Autodesk Inventor part; units mm, degrees
ref_plane "YZ Plane" through (0, 0, 0) normal (1, 0, 0) x (0, 1, 0)
ref_plane "XZ Plane" through (0, 0, 0) normal (0, 1, 0) x (-1, 0, 0)
ref_plane "XY Plane" through (0, 0, 0) normal (0, 0, 1) x (1, 0, 0)
sketch "Sketch2" plane through (0, 0, 0) normal (0, 0, 1) x (1, 0, 0)
  circle A0 centre (0, 0) radius 80.5
  circle A1 centre (0, 0) radius 142.5
  dimension "d25" = 161
  dimension "d27" = 285
extrude "Plate2" add sketch "Sketch2" along normal blind 8 contours A0 | A1
sketch "Sketch3" plane through (0, 0, 8) normal (0, 0, 1) x (1, 0, 0)
  circle A0 centre (-120, 0) radius 8.5
  circle A1 centre (0, 0) radius 120 construction
  dimension "d28" = 240
  dimension "d15" = 17
extrude "Cut1" cut sketch "Sketch3" against normal blind 8
pattern_circular "Circular Pattern1" count 8 over 360 about axis through (0, 0, -10) along (0, 0, 1) of "Cut1"
equation "\"d17\" = Thickness"
equation "\"d14\" = Thickness"
equation "\"BendReliefWidth\" = Thickness"
equation "\"BendReliefDepth\" = 0.5 * Thickness"
equation "\"CornerReliefSize\" = 4 * Thickness"
equation "\"MinimumRemnant\" = 2 * Thickness"
equation "\"TransitionRadius\" = BendRadius"
equation "\"JacobiRadiusSize\" = BendRadius"
equation "\"GapSize\" = Thickness"
properties part number "SLM 1707 charging flange cup" material "Steel"
Could you check a few things on this model? Use its own coordinates, in mm. Give positions to 0.01 mm unless a question says otherwise; leave off trailing zeros. Write each loop counter-clockwise with the first axis right and the second up, starting at its lowest first coordinate (ties: lowest second). Pieces come first, ordered by that corner, then holes. Notation, with made-up numbers: (77, 11.25) - (111, 11.25) arc R7 cw to (111, 18.25) - close; hole circle Ø3 at (46.25, 78.5). An arc over 180 degrees is marked (long way). One line per item, written item: value. Start each with the question number.
Item 1: Imagine slicing it at A-A, the plane y = 0. List the corners of the cut face in (x, z) for me, and give its area (3 significant figures).
Item 2: Please list where these lines run through material, in increasing order: line 1 (X direction, y = 87, z = 4.25); line 2 (X direction, y = 83, z = 4.25); line 3 (X direction, y = 114.5, z = 1.75). Write a range as from..to.
Item 3: Imagine slicing it at C-C, the plane y = 120. List the corners of the cut face in (x, z) for me.
Item 4: If we mould it in two halves opening along Y, with no side actions, what happens to faces 1 (the face through (-77, -81.6, 4.1)), 2 (the face through (-2, 2, 0)), 3 (the face through (-105.028, -96.308, 3.944)), 4 (the face through (-111.89, 2.55, 4.06))? For each: +Y half, -Y half, draft (parallel to the pull), parting line (faces both ways), or undercut.
Item 5: I'm going to push flat-ended pins straight in: pin 1 (13.5 mm diameter, centred on x = 84.85, y = 84.85, fed in from -Z); pin 2 (1.5 mm diameter, centred on x = 97.5, z = 2.5, fed in from +Y); pin 3 (2 mm diameter, centred on y = 55, z = 6, fed in from -X); pin 4 (3 mm diameter, centred on y = -69.5, z = 3, fed in from +X). Where does each tip first touch, or does it pass through?
Geometry says:
1. outline: (-142.5, 0) - (-128.5, 0) - (-128.5, 8) - (-142.5, 8) - close; (-111.5, 0) - (111.5, 0) - (111.5, 8) - (-111.5, 8) - close; (128.5, 0) - (142.5, 0) - (142.5, 8) - (128.5, 8) - close
1. area: 2,010 mm^2
2. line 1: -112.86..-93.08, -76.63..76.63, 93.08..112.86
2. line 2: -115.83..-93.15, -76.56..76.56, 93.15..115.83
2. line 3: -84.83..-6.48, 6.48..84.83
3. outline: (-76.85, 0) - (-8.5, 0) - (-8.5, 8) - (-76.85, 8) - close; (8.5, 0) - (76.85, 0) - (76.85, 8) - (8.5, 8) - close
4. face 1: undercut
4. face 2: draft
4. face 3: parting line
4. face 4: undercut
5. pin 1: through
5. pin 2: y = 104.62
5. pin 3: x = -131.87
5. pin 4: x = 125.23
